```python
from build123d import *

# Parameters (mm, degrees)
ESQUISSE1_W             = 10.15
ESQUISSE1_H             = 5
ENL_V_MAT_EXTRU_1_DEPTH = 1.9
TROU_TARAUD_M81_D       = 6.8
TROU_TARAUD_M81_DEPTH   = 22.25
TROU_TARAUD_M81_TIP     = 2.042926105


with BuildPart() as part:
    # Esquisse1 → Révolution1 (revolve)
    with BuildSketch(Plane.XY, mode=Mode.PRIVATE) as r_volution1_sk:
        with Locations((-7.575, 2.5)):
            Rectangle(ESQUISSE1_W, ESQUISSE1_H)
    revolve(r_volution1_sk.sketch.rotate(Axis((0, 0, 0), (0, 1, 0)), 270), axis=Axis((0, 0, 0), (0, 1, 0)))

    # Esquisse2 → Enlèv. mat.-Extru.1 (cut)
    with BuildSketch(Plane(origin=(0, 5, 0), x_dir=(1, 0, 0), z_dir=(0, 1, 0))):
        with BuildLine():
            Line((-2.5, 12.400504022), (-2.5, -12.400504022))
            ThreePointArc((-2.5, -12.400504022), (0, -12.65), (2.5, -12.400504022))
            Line((2.5, -12.400504022), (2.5, 12.400504022))
            ThreePointArc((2.5, 12.400504022), (0, 12.65), (-2.5, 12.400504022))
        make_face()
    extrude(amount=-ENL_V_MAT_EXTRU_1_DEPTH, mode=Mode.SUBTRACT)

    # Trou taraudé M81
    with Locations(Plane.XZ):
        with Locations((0, 0)):
            Hole(TROU_TARAUD_M81_D / 2, depth=TROU_TARAUD_M81_DEPTH)
            with Locations((0, 0, -(TROU_TARAUD_M81_DEPTH + TROU_TARAUD_M81_TIP / 2))):  # 118° drill point
                Cone(0, TROU_TARAUD_M81_D / 2, TROU_TARAUD_M81_TIP, mode=Mode.SUBTRACT)


solid = part.part
```
The listing builds one solid part. Answer for the finished solid, in the listing's coordinates (mm). A direction names the side the tool comes from. Give positions to 0.01 mm unless a question says otherwise; leave off trailing zeros. Order: outer loops, then holes, each group sorted by start corner. A loop starts at its lowest first (then second) coordinate and runs counter-clockwise, first axis right, second up.
1) Find section B-B on x = 0. Write down the section's boundary in (y, z).
Reported:
outline: (0, -12.65) - (3.1, -12.65) - (3.1, -3.4) - (0, -3.4) - close; (0, 3.4) - (3.1, 3.4) - (3.1, 12.65) - (0, 12.65) - close
2) Find section A-A on z = 0. Write down the section's boundary in (x, y), then the cut area to 3 significant figures.
Reported:
outline: (-12.65, 0) - (-3.4, 0) - (-3.4, 5) - (-12.65, 5) - close; (3.4, 0) - (12.65, 0) - (12.65, 5) - (3.4, 5) - close
area: 92.5 mm2
3) Given P1, Ø1.5, axis at y = 4, z = 9.5, coming from the +X side; P2, Ø5.5, axis at x = 0, z = 0, coming from the -Y side; P3, Ø1, axis at y = 4.5, z = 8.5, coming from the -X side; P4, Ø1.5, axis at y = 4, z = -9, coming from the +X side, each flat-ended and moving along its own axis, determine where each tip first touches the part or whether it passes through.
Reported:
P1: stops at x = 9.14
P2: passes through
P3: stops at x = -9.8
P4: stops at x = 9.59
4) Determine the mould class of faces 3 (the face through (-7, 5, 0)), 4 (the face through (-2.5, 4, -7)), 5 (the face through (-4, 3, -12)) for opening direction X: pulls with the +X half, pulls with the -X half, needs draft (parallel to the pull), parting line crosses it, or undercut.
Reported:
face 3: needs draft
face 4: undercut
face 5: parting line crosses it
5) Find section D-D on y = 0.8. Write down the section's boundary in (x, z), then the cut area to 3 significant figures.
Reported:
outline: circle Ø25.3 at (0, 0); hole circle Ø6.8 at (0, 0)
area: 466 mm2
6) Consider line 1 along X through (y, z) = (3.4, 0); line 2 along X through (y, z) = (1.5, -2.5); line 3 along Z through (x, y) = (1.25, 1.8). Determine where each line is inside the solid, lowest interval first.
Reported:
line 1: x = -12.65 to -3.4, 3.4 to 12.65
line 2: x = -12.4 to -2.3, 2.3 to 12.4
line 3: z = -12.59 to -3.16, 3.16 to 12.59
7) For faces 1 (the face through (3, 0, -3)), 2 (the face through (2.5, 4, -7)), determine the directions among +Z, -Z, +X, -X, +Y, -Y from which every point of the face is accessible in a straight line to the end or side of a thin tool.
Reported:
face 1: +Z, -Z, +X, -X, -Y
face 2: +Z, -Z, +Y
8) Find section C-C on z = 5. Write down the section's boundary in (x, y).
Reported:
outline: (-11.62, 0) - (11.62, 0) - (11.62, 5) - (2.5, 5) - (2.5, 3.1) - (-2.5, 3.1) - (-2.5, 5) - (-11.62, 5) - close
